from build123d import *

# Parameters (mm, degrees)
BOSS_EXTRUDE1_DEPTH        = 12.7508
SHELL2_T                   = -3.81
F_50_0_07_DIAMETER_HOLE3_D = 1.778
SKETCH15_R                 = 3.99415
CUT_EXTRUDE2_DEPTH         = 85.623521635
SKETCH16_R                 = 2.39395
CUT_EXTRUDE3_DEPTH         = 85.623521635


with BuildPart() as part:
    # Sketch1 → Boss-Extrude1 (new body)
    with BuildSketch(Plane.XY):
        with BuildLine():
            Line((0, 0), (31.187102024, -17.823710818))
            ThreePointArc((31.187102024, -17.823710818), (53.082286429, -15.709260563), (58.387158413, 5.638534012))
            Line((58.387158413, 5.638534012), (45.333427314, 39.103741383))
            ThreePointArc((45.333427314, 39.103741383), (-4.983807045, 51.60744456), (0, 0))
        make_face()
    extrude(amount=BOSS_EXTRUDE1_DEPTH)

    # Shell2
    shell2_openings = [part.faces().sort_by_distance(p)[0] for p in [
        (22.133833563, 20.169644853, 12.7508),
    ]]
    offset(amount=SHELL2_T, openings=shell2_openings, kind=Kind.INTERSECTION)

    # #50 (0.07) Diameter Hole3 (through all)
    with Locations(Plane.XY.offset(12.7508)):
        with Locations((-3.770169746, 50.098384989), (14.127303317, 57.178704003), (37.679197815, 48.033291943), (57.887608334, 0.388645245), (52.380693545, -13.624486137), (33.69651837, -16.967970116), (9.898779461, -3.544865319), (-4.606040741, 5.748053387), (-13.01391957, 20.154535826), (-12.52223075, 37.166969012), (44.661179065, 35.741071433), (53.265733422, 13.860918924)):
            Hole(F_50_0_07_DIAMETER_HOLE3_D / 2)

    # Sketch15 → Cut-Extrude2 (cut, through all)
    with BuildSketch(Plane.XY.offset(3.81)):
        with Locations((15.754083482, 27.565764159)):
            Circle(SKETCH15_R)
    extrude(amount=-CUT_EXTRUDE2_DEPTH, mode=Mode.SUBTRACT)

    # Sketch16 → Cut-Extrude3 (cut, through all)
    with BuildSketch(Plane.XY.offset(3.81)):
        with Locations((27.159923271, 14.342839938)):
            Circle(SKETCH16_R)
    extrude(amount=-CUT_EXTRUDE3_DEPTH, mode=Mode.SUBTRACT)


solid = part.part
Can you work these out from the model? Positions are in its coordinate system, mm. A direction names the side the tool comes from. Give positions to 0.01 mm unless a question says otherwise; leave off trailing zeros. Order: outer loops, then holes, each group sorted by start corner. A loop starts at its lowest first (then second) coordinate and runs counter-clockwise, first axis right, second up. Notation, with made-up numbers: (48.5, -9) - (100.5, -9) arc R11 ccw to (100.5, -2) - close; hole circle Ø7 at (-6, -2). An arc over 180 degrees is marked (long way). Write each question's results on one line, items separated by ' | '.
1) If we mould it in two halves opening along Y, with no side actions, what happens to faces 3 (the face through (15.4, -8.8, 6.3)), 4 (the face through (21, 20, 0)), 5 (the face through (57.04, 0.66, 6.29)), 6 (the face through (-1.923, 49.203, 8.218))? For each: pulls with the +Y half, pulls with the -Y half, needs draft (parallel to the pull), parting line crosses it, or undercut.
Final values:
face 3: pulls with the -Y half | face 4: needs draft | face 5: undercut | face 6: undercut
2) Suppose I cut it at A-A, the plane x = 26. Write out the boundary of the cut face in (y, z).
Final values:
outline: (-14.86, 0) - (12.25, 0) - (12.25, 3.81) - (-10.47, 3.81) - (-10.47, 12.75) - (-14.86, 12.75) - close; (16.44, 0) - (57.62, 0) - (57.62, 12.75) - (53.56, 12.75) - (53.56, 3.81) - (16.44, 3.81) - close
3) On a 3-axis mill with a long thin cutter (end or side, diameter ignored), from which of +Z, -Z, +X, -X, +Y, -Y can I reach the whole of each face in a straight line? I mean faces 1 (the face through (48.402, 20.752, 8.218)), 2 (the face through (34.585, -16.929, 6.286)). Say none if no direction works.
Final values:
face 1: +Z | face 2: +Z, -Z
4) I'm going to push flat-ended pins straight in: pin 1 Ø3 at (y, z) = (17, 6.5) entering from -X; pin 2 Ø6 at (x, z) = (33, 5) entering from +Y; pin 3 Ø2 at (y, z) = (18, 4.5) entering from -X. Where does each tip first touch, or does it pass through?
Final values:
pin 1: stops at x = -14.67 | pin 2: stops at y = 55.94 | pin 3: stops at x = -14.82
5) Suppose I cut it at C-C, the plane y = 25. Write out the boundary of the cut face in (x, z).
Final values:
outline: (-15.89, 0) - (12.69, 0) - (12.69, 3.81) - (-12.07, 3.81) - (-12.07, 12.75) - (-15.89, 12.75) - close; (18.82, 0) - (50.83, 0) - (50.83, 12.75) - (46.75, 12.75) - (46.75, 3.81) - (18.82, 3.81) - close
6) Suppose I cut it at D-D, the plane x = -8.5. Write out the boundary of the cut face in (y, z), then the cut area to 3 significant figures.
Final values:
outline: (7.08, 0) - (48.05, 0) - (48.05, 12.75) - (41.44, 12.75) - (41.44, 3.81) - (13.7, 3.81) - (13.7, 12.75) - (7.08, 12.75) - close | area: 274 mm^2
7) Suppose I cut it at B-B, the plane z = 4.75. Give the number of separate pieces and of enclosed holes in the cut face, then the cut area to 3 significant figures.
Final values:
separate pieces: 1 | enclosed holes: 13 | area: 839 mm^2
8) Please list where these lines run through material, in increasing order: line 1 along Y through (x, z) = (34.5, 5.5); line 2 along Z through (x, y) = (4, 43); line 3 along X through (y, z) = (37.5, 5.5). Write a range as [from, to].
Final values:
line 1: y = [-19.32, -17.35], [-16.59, -15.23], [48.28, 53.19] | line 2: z = [0, 3.81] | line 3: x = [-14.4, -13.35], [-11.7, -10.36], [41.87, 45.96]
